Read the model definition and answer for the solid it produces. Units are mm, in the model's axes. Round coordinates to 2 decimals unless told otherwise and drop trailing zeros. Order: outer loops, then holes, each group sorted by start corner. A loop starts at its lowest first (then second) coordinate and runs counter-clockwise, first axis right, second up. Notation, with made-up numbers: (-31, 18) -> (24, 18) arc R21 cw to (24, 22) -> close; hole circle Ø4 at (1, 55.25). An arc over 180 degrees is marked (long way). One line per item, written item: value. Start each with the question number.
1. Consider line 1 (X direction, y = 3.75, z = 0.45); line 2 (X direction, y = 4, z = 0.4). Determine where each line is inside the solid, lowest interval first.
2. A flat-ended cylindrical pin translates along its axis: pin 1 Ø8 at (x, y) = (0, 0) entering from +Z. Find the tip coordinate at first contact, or state that the pin passes through.
3. Section B-B (x = 0) is taken. Give the vertices of the cut face in (y, z), then the cut area to 3 significant figures.
4. Section A-A (x = 6) is taken. Give the vertices of the cut face in (y, z).
from build123d import *

# Parameters (mm, degrees)
SKETCH_1_R      = 7.5
SKETCH_1_R_2    = 1.15
SKETCH_1_R_3    = 4.5
EXTRUDE_1_DEPTH = 0.5


with BuildPart() as part:
    # 草图1 → 凸台-拉伸1 (new body)
    with BuildSketch(Plane.XY):
        Circle(SKETCH_1_R)
        with Locations((0, 6)):
            Circle(SKETCH_1_R_2, mode=Mode.SUBTRACT)
        Circle(SKETCH_1_R_3, mode=Mode.SUBTRACT)
        with Locations((4.242640687, 4.242640687)):
            Circle(SKETCH_1_R_2, mode=Mode.SUBTRACT)
        with Locations((6, 0)):
            Circle(SKETCH_1_R_2, mode=Mode.SUBTRACT)
        with Locations((4.242640687, -4.242640687)):
            Circle(SKETCH_1_R_2, mode=Mode.SUBTRACT)
        with Locations((0, -6)):
            Circle(SKETCH_1_R_2, mode=Mode.SUBTRACT)
        with Locations((-4.242640687, -4.242640687)):
            Circle(SKETCH_1_R_2, mode=Mode.SUBTRACT)
        with Locations((-6, 0)):
            Circle(SKETCH_1_R_2, mode=Mode.SUBTRACT)
        with Locations((-4.242640687, 4.242640687)):
            Circle(SKETCH_1_R_2, mode=Mode.SUBTRACT)
    extrude(amount=EXTRUDE_1_DEPTH)


solid = part.part
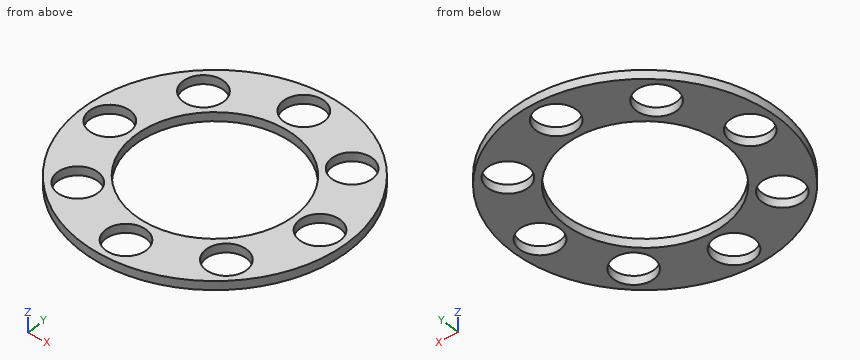
Answer:
1. line 1: -6.5 to -5.28, -3.2 to -2.49, 2.49 to 3.2, 5.28 to 6.5
1. line 2: -6.34 to -5.37, -3.12 to -2.06, 2.06 to 3.12, 5.37 to 6.34
2. pin 1: through
3. outline: (-7.5, 0) -> (-7.15, 0) -> (-7.15, 0.5) -> (-7.5, 0.5) -> close; (-4.85, 0) -> (-4.5, 0) -> (-4.5, 0.5) -> (-4.85, 0.5) -> close; (4.5, 0) -> (4.85, 0) -> (4.85, 0.5) -> (4.5, 0.5) -> close; (7.15, 0) -> (7.5, 0) -> (7.5, 0.5) -> (7.15, 0.5) -> close
3. area: 0.700 mm^2
4. outline: (-4.5, 0) -> (-1.15, 0) -> (-1.15, 0.5) -> (-4.5, 0.5) -> close; (1.15, 0) -> (4.5, 0) -> (4.5, 0.5) -> (1.15, 0.5) -> close
